from build123d import *

# Parameters (mm, degrees)
MODEL_R             = 1.375
MODEL_W             = 14
MODEL_H             = 5.35
MODEL_W_2           = 5.35
MODEL_H_2           = 11
BOSS_EXTRUDE1_DEPTH = 5.35


with BuildPart() as part:
    # Model → Boss-Extrude1 (new body)
    with BuildSketch(Plane.XY):
        Polygon((0, 0), (58, 0), (58, 5.35), (64, 5.35), (64, 21.55), (58, 21.55), (58, 26.9), (64, 26.9), (64, 43.1), (58, 43.1), (58, 48.45), (64, 48.45), (64, 64.65), (58, 64.65), (58, 70), (0, 70), (0, 64.65), (-6, 64.65), (-6, 48.45), (0, 48.45), (0, 43.1), (-6, 43.1), (-6, 26.9), (0, 26.9), (0, 21.55), (-6, 21.55), (-6, 5.35), (0, 5.35), align=None)
        with Locations((-3, 56.55)):
            Circle(MODEL_R, mode=Mode.SUBTRACT)
        with Locations(Location((61, 56.55, 0), (0, 0, 180))):
            Circle(MODEL_R, mode=Mode.SUBTRACT)
        with Locations((61, 13.45)):
            Circle(MODEL_R, mode=Mode.SUBTRACT)
        with Locations(Location((-3, 13.45, 0), (0, 0, 180))):
            Circle(MODEL_R, mode=Mode.SUBTRACT)
        with Locations((-3, 35)):
            Circle(MODEL_R, mode=Mode.SUBTRACT)
        with Locations(Location((61, 35, 0), (0, 0, 180))):
            Circle(MODEL_R, mode=Mode.SUBTRACT)
        with Locations((15, 62.155)):
            Rectangle(MODEL_W, MODEL_H, mode=Mode.SUBTRACT)
        with Locations((43, 62.155)):
            Rectangle(MODEL_W, MODEL_H, mode=Mode.SUBTRACT)
        with Locations((43, 7.845)):
            Rectangle(MODEL_W, MODEL_H, mode=Mode.SUBTRACT)
        with Locations((15, 7.845)):
            Rectangle(MODEL_W, MODEL_H, mode=Mode.SUBTRACT)
        with Locations((16.325, 35)):
            Rectangle(MODEL_W_2, MODEL_H_2, mode=Mode.SUBTRACT)
        with Locations((41.675, 35)):
            Rectangle(MODEL_W_2, MODEL_H_2, mode=Mode.SUBTRACT)
    extrude(amount=BOSS_EXTRUDE1_DEPTH)


solid = part.part
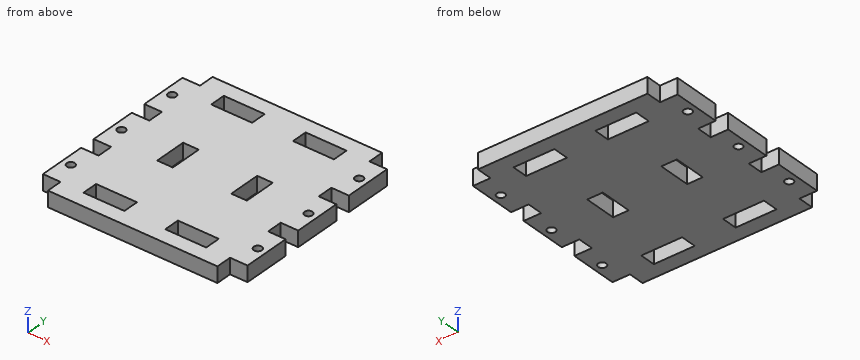
The model under review builds one solid part; all positions refer to its coordinate system, in mm. Give positions to 0.01 mm unless a question says otherwise; leave off trailing zeros. Loops run counter-clockwise (first coordinate to the right, second up) from the corner with the lowest first, then second, coordinate; pieces in that order, holes last. Notation, with made-up numbers: (49.25, 13.25) -> (84.25, 13.25) arc R11 cw to (84.25, 26.25) -> close; hole circle Ø6 at (14, -8). An arc over 180 degrees is marked (long way). Answer as a JSON object with one key per item and string values. Group by question number.
Q1. Insertion check: pin 1 (1.6 mm diameter, centred on y = 25, z = 2.5, fed in from +X). The pin has a flat end and moves straight along its axis. Give the tip position at first contact, or say it passes through.
Q2. Take a section at D-D (x = 61). Write out the cut boundary in (y, z) (3 decimals), plus the area to 3 significant figures.
Q3. Wall thickness on line 1 along X through (y, z) = (61, 2.3); line 2 along Y through (x, z) = (-3, 3.4) (3 decimals); line 3 along Y through (x, z) = (19.5, 4.35): over which ranges is each line inside the solid? List them lowest first.
Q4. Take a section at C-C (y = 56.55). Write out the cut boundary in (x, z) (3 decimals).
Q5. Take a section at A-A (x = 42.5). Write out the cut boundary in (y, z).
Q6. Take a section at B-B (y = 35). Write out the cut boundary in (x, z) (3 decimals).
Answer below:
{
 "1": {"pin 1": "stops at x = 58"},
 "2": {"outline": "(5.35, 0) -> (12.075, 0) -> (12.075, 5.35) -> (5.35, 5.35) -> close; (14.825, 0) -> (21.55, 0) -> (21.55, 5.35) -> (14.825, 5.35) -> close; (26.9, 0) -> (33.625, 0) -> (33.625, 5.35) -> (26.9, 5.35) -> close; (36.375, 0) -> (43.1, 0) -> (43.1, 5.35) -> (36.375, 5.35) -> close; (48.45, 0) -> (55.175, 0) -> (55.175, 5.35) -> (48.45, 5.35) -> close; (57.925, 0) -> (64.65, 0) -> (64.65, 5.35) -> (57.925, 5.35) -> close", "area": "216 mm2"},
 "3": {"line 1": "x = -6 to 8, 22 to 36, 50 to 64", "line 2": "y = 5.35 to 12.075, 14.825 to 21.55, 26.9 to 33.625, 36.375 to 43.1, 48.45 to 55.175, 57.925 to 64.65", "line 3": "y = 0 to 5.17, 10.52 to 59.48, 64.83 to 70"},
 "4": {"outline": "(-6, 0) -> (-4.375, 0) -> (-4.375, 5.35) -> (-6, 5.35) -> close; (-1.625, 0) -> (59.625, 0) -> (59.625, 5.35) -> (-1.625, 5.35) -> close; (62.375, 0) -> (64, 0) -> (64, 5.35) -> (62.375, 5.35) -> close"},
 "5": {"outline": "(0, 0) -> (5.17, 0) -> (5.17, 5.35) -> (0, 5.35) -> close; (10.52, 0) -> (29.5, 0) -> (29.5, 5.35) -> (10.52, 5.35) -> close; (40.5, 0) -> (59.48, 0) -> (59.48, 5.35) -> (40.5, 5.35) -> close; (64.83, 0) -> (70, 0) -> (70, 5.35) -> (64.83, 5.35) -> close"},
 "6": {"outline": "(-6, 0) -> (-4.375, 0) -> (-4.375, 5.35) -> (-6, 5.35) -> close; (-1.625, 0) -> (13.65, 0) -> (13.65, 5.35) -> (-1.625, 5.35) -> close; (19, 0) -> (39, 0) -> (39, 5.35) -> (19, 5.35) -> close; (44.35, 0) -> (59.625, 0) -> (59.625, 5.35) -> (44.35, 5.35) -> close; (62.375, 0) -> (64, 0) -> (64, 5.35) -> (62.375, 5.35) -> close"}
}
